from build123d import *

# Parameters (mm, degrees)
BOSS_EXTRUDE1_DEPTH      = 17
SKETCH10_W               = 3
SKETCH10_H               = 4
SKETCH10_H_2             = 2
BOSS_EXTRUDE8_DEPTH      = 0.4
SKETCH11_W               = 2
SKETCH11_H               = 2.1
SKETCH11_W_2             = 4
BOSS_EXTRUDE9_DEPTH      = 0.4
FILLET5_R                = 0.4
SPLIT2_SURFACE_1_BACK    = 26.421
SPLIT2_SURFACE_1_DEPTH   = 52.842
SPLIT2_SURFACE_2_BACK    = 26.421
SPLIT2_SURFACE_2_DEPTH   = 52.842
FILLET6_R                = 1.5
SKETCH13_W               = 5.8
SKETCH13_H               = 8.5
BOSS_EXTRUDE10_DEPTH     = 3
FILLET7_R                = 4
SPLIT3_SURFACE_3_BACK    = 34.598
SPLIT3_SURFACE_3_DEPTH   = 69.196
SPLIT3_SURFACE_4_BACK    = 34.598
SPLIT3_SURFACE_4_DEPTH   = 69.196
CUT_EXTRUDE1_DEPTH       = 1.5
CUT_EXTRUDE2_DEPTH       = 29.664263465
DELETEFACE1_START        = 1.5
DELETEFACE1_DEPTH        = 12
CUT_EXTRUDE3_DEPTH       = 8
MOVE_START               = 1.5
MOVE_FACE1_OUTLINE_W     = 2.5
MOVE_FACE1_OUTLINE_H     = 4
MOVE_FACE1_OUTLINE_H_2   = 2
MOVE_FACE1_DEPTH         = 3
MOVE_FACE1_2_OUTLINE_W   = 0.4
MOVE_FACE1_2_OUTLINE_H   = 2
MOVE_FACE1_2_OUTLINE_H_2 = 4
MOVE_FACE1_2_DEPTH       = 3
MOVE_FACE1_3_OUTLINE_W   = 2.1
MOVE_FACE1_3_OUTLINE_H   = 2
MOVE_FACE1_3_OUTLINE_H_2 = 4
MOVE_FACE1_3_DEPTH       = 0.4
CUT_EXTRUDE4_DEPTH       = 25.456900867
CUT_EXTRUDE4_DEPTH_BACK  = 25.456900867
SPLIT4_SURFACE_5_BACK    = 32.215
SPLIT4_SURFACE_5_DEPTH   = 64.43
SPLIT4_SURFACE_6_BACK    = 32.215
SPLIT4_SURFACE_6_DEPTH   = 64.43
FILLET8_R                = 1
MOVE_START_2             = 1.35
MOVE_FACE2_DEPTH         = 0.15
MOVE_START_3             = 3.2
MOVE_FACE2_2_DEPTH       = 0.15
SPLIT5_START             = -5.8
SPLIT5_OUTLINE_W         = 3
SPLIT5_OUTLINE_H         = 8.5
SPLIT5_DEPTH             = 5.8
SPLIT5_START_2           = 15
SPLIT5_2_OUTLINE_W       = 3
SPLIT5_2_OUTLINE_H       = 8.5
SPLIT5_2_DEPTH           = 5.8
DELETEFACE2_DEPTH        = 1.5
DELETEFACE2_START        = 13.5
DELETEFACE2_2_DEPTH      = 1.5


# Read off the part's stored shape, not the designer's step: DeleteFace1, Move Face1, Move Face2, Split5, DeleteFace2
with BuildPart() as part:
    # Sketch1 → Boss-Extrude1 (new body)
    with BuildSketch(Plane.XY):
        Polygon((0, 0), (1.5, 0), (1.5, 10), (13.5, 10), (13.5, 0), (15, 0), (15, 11.5), (0, 11.5), (0, 10), align=None)
    extrude(amount=BOSS_EXTRUDE1_DEPTH)

    # Sketch10 → Boss-Extrude8 (add)
    with BuildSketch(Plane.XZ.offset(-10)):
        with Locations((12, 14)):
            Rectangle(SKETCH10_W, SKETCH10_H)
        with Locations((12, 10)):
            Rectangle(SKETCH10_W, SKETCH10_H_2)
    boss_extrude8 = extrude(amount=BOSS_EXTRUDE8_DEPTH)

    # Sketch11 → Boss-Extrude9 (add)
    with BuildSketch(Plane.ZY.offset(-13.5)):
        with Locations((10, 8.55)):
            Rectangle(SKETCH11_W, SKETCH11_H)
        with Locations((14, 8.55)):
            Rectangle(SKETCH11_W_2, SKETCH11_H)
    boss_extrude9 = extrude(amount=BOSS_EXTRUDE9_DEPTH)

    # Fillet5
    fillet5_edges = [part.edges().sort_by_distance(p)[0] for p in [
        (13.1, 9.6, 10),
        (13.1, 9.6, 14),
    ]]
    fillet(fillet5_edges, radius=FILLET5_R)


with BuildPart() as body_2:
    # Split2: the piece behind the surface
    add(part.part)
    # Split2 surface: a surface, the sketch's curves swept straight by 52.842 mm
    with BuildLine(Plane.XZ.offset(-SPLIT2_SURFACE_1_BACK), mode=Mode.PRIVATE) as split2_surface_1_path:
        Line((15, 8), (0, 8))
    split2_surface_1 = Shell.extrude(split2_surface_1_path.wire(), (0 * SPLIT2_SURFACE_1_DEPTH, -1 * SPLIT2_SURFACE_1_DEPTH, 0 * SPLIT2_SURFACE_1_DEPTH))
    split(bisect_by=split2_surface_1, keep=Keep.BOTTOM)


with BuildPart() as part_1:
    add(part.part)

    # Split2: split by a surface, the side it looks to stays
    # Split2 surface: a surface, the sketch's curves swept straight by 52.842 mm
    with BuildLine(Plane.XZ.offset(-SPLIT2_SURFACE_2_BACK), mode=Mode.PRIVATE) as split2_surface_2_path:
        Line((15, 8), (0, 8))
    split2_surface_2 = Shell.extrude(split2_surface_2_path.wire(), (0 * SPLIT2_SURFACE_2_DEPTH, -1 * SPLIT2_SURFACE_2_DEPTH, 0 * SPLIT2_SURFACE_2_DEPTH))
    split(bisect_by=split2_surface_2, keep=Keep.TOP)

    # Fillet6
    fillet6_edges = [part_1.edges().sort_by_distance(p)[0] for p in [
        (13.5, 10, 4),
        (1.5, 10, 4),
    ]]
    fillet(fillet6_edges, radius=FILLET6_R)


with BuildPart() as body_2_1:
    add(body_2.part)

    # Combine2: union part
    add(part_1.part)

    # Sketch13 → Boss-Extrude10 (add)
    with BuildSketch(Plane.XZ):
        with Locations((-2.9, 4.25)):
            Rectangle(SKETCH13_W, SKETCH13_H)
        with Locations((17.9, 4.25)):
            Rectangle(SKETCH13_W, SKETCH13_H)
    extrude(amount=-BOSS_EXTRUDE10_DEPTH)

    # Fillet7
    fillet7_edges = [body_2_1.edges().sort_by_distance(p)[0] for p in [
        (20.8, 1.5, 8.5),
        (20.8, 1.5, 0),
        (-5.8, 1.5, 0),
        (-5.8, 1.5, 8.5),
    ]]
    fillet(fillet7_edges, radius=FILLET7_R)


with BuildPart() as body_2_2:
    # Split3: the piece behind the surface
    add(body_2_1.part)
    # Split3 surface: a surface, the sketch's curves swept straight by 69.196 mm
    with BuildLine(Plane.ZY.offset(-SPLIT3_SURFACE_3_BACK), mode=Mode.PRIVATE) as split3_surface_3_path:
        Line((0, 3), (17, 3))
    split3_surface_3 = Shell.extrude(split3_surface_3_path.wire(), (-1 * SPLIT3_SURFACE_3_DEPTH, 0 * SPLIT3_SURFACE_3_DEPTH, 0 * SPLIT3_SURFACE_3_DEPTH))
    split(bisect_by=split3_surface_3, keep=Keep.BOTTOM)

    # Sketch16 → Cut-Extrude1 (cut)
    with BuildSketch(Plane(origin=(0, 3, 0), x_dir=(1, 0, 0), z_dir=(0, 1, 0))):
        Polygon((-1, -7.136751346), (1.5, -5.693375673), (1.5, -2.806624327), (-1, -1.363248654), (-3.5, -2.806624327), (-3.5, -5.693375673), align=None)
        Polygon((16, -1.363248654), (13.5, -2.806624327), (13.5, -5.693375673), (16, -7.136751346), (18.5, -5.693375673), (18.5, -2.806624327), align=None)
    extrude(amount=-CUT_EXTRUDE1_DEPTH, mode=Mode.SUBTRACT)

    # Sketch17 → Cut-Extrude2 (cut, through all)
    with BuildSketch(Plane(origin=(0, 1.5, 0), x_dir=(1, 0, 0), z_dir=(0, 1, 0))):
        with BuildLine():
            Line((16, -5.25), (13.5, -5.25))
            Line((13.5, -5.25), (13.5, -3.25))
            Line((13.5, -3.25), (16, -3.25))
            ThreePointArc((16, -3.25), (17, -4.25), (16, -5.25))
        make_face()
        with BuildLine():
            Line((1.5, -3.25), (1.5, -5.25))
            Line((1.5, -5.25), (-1, -5.25))
            ThreePointArc((-1, -5.25), (-2, -4.25), (-1, -3.25))
            Line((-1, -3.25), (1.5, -3.25))
        make_face()
    extrude(amount=-CUT_EXTRUDE2_DEPTH, mode=Mode.SUBTRACT)


with BuildPart() as body_2_3:
    add(body_2_1.part)

    # Split3: split by a surface, the side it looks to stays
    # Split3 surface: a surface, the sketch's curves swept straight by 69.196 mm
    with BuildLine(Plane.ZY.offset(-SPLIT3_SURFACE_4_BACK), mode=Mode.PRIVATE) as split3_surface_4_path:
        Line((0, 3), (17, 3))
    split3_surface_4 = Shell.extrude(split3_surface_4_path.wire(), (-1 * SPLIT3_SURFACE_4_DEPTH, 0 * SPLIT3_SURFACE_4_DEPTH, 0 * SPLIT3_SURFACE_4_DEPTH))
    split(bisect_by=split3_surface_4, keep=Keep.TOP)

    # Combine3: union body 2 2
    add(body_2_2.part)

    # DeleteFace1 outline → DeleteFace1 (cut)
    with BuildSketch(Plane.YZ.offset(DELETEFACE1_START)):
        Polygon((10, -1), (10, 8), (10, 9), (7, 9), (7, -1), align=None)
    extrude(amount=DELETEFACE1_DEPTH, mode=Mode.SUBTRACT)

    # Mirror1: Boss-Extrude8, Boss-Extrude9 across plane
    add(boss_extrude8.mirror(Plane.ZY.offset(-7.5)))
    add(boss_extrude9.mirror(Plane.ZY.offset(-7.5)))

    # Sketch18 → Cut-Extrude3 (cut)
    with BuildSketch(Plane.XY.offset(16)):
        with BuildLine():
            Line((13.5, 10), (10.5, 10))
            Line((10.5, 10), (10.5, 9.6))
            Line((10.5, 9.6), (12.7, 9.6))
            ThreePointArc((12.7, 9.6), (12.982842712, 9.482842712), (13.1, 9.2))
            Line((13.1, 9.2), (13.1, 7.5))
            Line((13.1, 7.5), (13.5, 7.5))
            Line((13.5, 7.5), (13.5, 10))
        make_face()
    extrude(amount=-CUT_EXTRUDE3_DEPTH, mode=Mode.SUBTRACT)

    # Move Face1 outline → Move Face1 (cut)
    with BuildSketch(Plane.YZ.offset(MOVE_START)):
        with Locations((8.75, 14)):
            Rectangle(MOVE_FACE1_OUTLINE_W, MOVE_FACE1_OUTLINE_H)
        with Locations((8.75, 10)):
            Rectangle(MOVE_FACE1_OUTLINE_W, MOVE_FACE1_OUTLINE_H_2)
    extrude(amount=MOVE_FACE1_DEPTH, mode=Mode.SUBTRACT)

    # Move Face1 2 outline → Move Face1 2 (add)
    with BuildSketch(Plane.YZ.offset(MOVE_START)):
        with Locations((9.8, 2.35)):
            Rectangle(MOVE_FACE1_2_OUTLINE_W, MOVE_FACE1_2_OUTLINE_H)
        with Locations((9.8, 6.35)):
            Rectangle(MOVE_FACE1_2_OUTLINE_W, MOVE_FACE1_2_OUTLINE_H_2)
    extrude(amount=MOVE_FACE1_2_DEPTH)

    # Move Face1 3 outline → Move Face1 3 (add)
    with BuildSketch(Plane.YZ.offset(MOVE_START)):
        with Locations((8.55, 2.35)):
            Rectangle(MOVE_FACE1_3_OUTLINE_W, MOVE_FACE1_3_OUTLINE_H)
        with Locations((8.55, 6.35)):
            Rectangle(MOVE_FACE1_3_OUTLINE_W, MOVE_FACE1_3_OUTLINE_H_2)
    extrude(amount=MOVE_FACE1_3_DEPTH)

    # Sketch19 → Cut-Extrude4 (cut, two sides: drawn at the far end of the back side and taken through both)
    with BuildSketch(Plane.ZY.offset(-7.5).offset(-CUT_EXTRUDE4_DEPTH_BACK)):
        Polygon((11.6, 62.452218571), (11.6, 13.786177198), (11.6, -3.966275857), (11.6, -52.632317231), (108.932082748, -52.632317231), (108.932082748, 62.452218571), align=None)
    extrude(amount=CUT_EXTRUDE4_DEPTH + CUT_EXTRUDE4_DEPTH_BACK, mode=Mode.SUBTRACT)


with BuildPart() as body_2_3_1:
    # Split4: the piece behind the surface
    add(body_2_3.part)
    # Split4 surface: a surface, the sketch's curves swept straight by 64.43 mm
    with BuildLine(Plane.ZY.offset(-7.5).offset(-SPLIT4_SURFACE_5_BACK), mode=Mode.PRIVATE) as split4_surface_5_path:
        Line((9.853674878, 13.930908587), (9.853674878, -3.706091584))
    split4_surface_5 = Shell.extrude(split4_surface_5_path.wire(), (-1 * SPLIT4_SURFACE_5_DEPTH, 0 * SPLIT4_SURFACE_5_DEPTH, 0 * SPLIT4_SURFACE_5_DEPTH))
    split(bisect_by=split4_surface_5, keep=Keep.BOTTOM)


with BuildPart() as body_2_4:
    add(body_2_3.part)

    # Split4: split by a surface, the side it looks to stays
    # Split4 surface: a surface, the sketch's curves swept straight by 64.43 mm
    with BuildLine(Plane.ZY.offset(-7.5).offset(-SPLIT4_SURFACE_6_BACK), mode=Mode.PRIVATE) as split4_surface_6_path:
        Line((9.853674878, 13.930908587), (9.853674878, -3.706091584))
    split4_surface_6 = Shell.extrude(split4_surface_6_path.wire(), (-1 * SPLIT4_SURFACE_6_DEPTH, 0 * SPLIT4_SURFACE_6_DEPTH, 0 * SPLIT4_SURFACE_6_DEPTH))
    split(bisect_by=split4_surface_6, keep=Keep.TOP)

    # Fillet8
    fillet8_edges = [body_2_4.edges().sort_by_distance(p)[0] for p in [
        (1.5, 10, 10.726837439),
        (13.5, 10, 10.726837439),
    ]]
    fillet(fillet8_edges, radius=FILLET8_R)

    # Combine4: union body 2 3
    add(body_2_3_1.part)

    # Move Face2 outline → Move Face2 (cut)
    with BuildSketch(Plane.XY.offset(MOVE_START_2)):
        Polygon((4.5, 10), (1.5, 10), (1.5, 7.5), (1.9, 7.5), (1.9, 9.6), (4.5, 9.6), align=None)
    extrude(amount=MOVE_FACE2_DEPTH, mode=Mode.SUBTRACT)

    # Move Face2 2 outline → Move Face2 2 (cut)
    with BuildSketch(Plane.XY.offset(MOVE_START_3)):
        Polygon((4.5, 10), (1.5, 10), (1.5, 7.5), (1.9, 7.5), (1.9, 9.6), (4.5, 9.6), align=None)
    extrude(amount=MOVE_FACE2_2_DEPTH, mode=Mode.SUBTRACT)

    # Split5 outline → Split5 (cut)
    with BuildSketch(Plane.YZ.offset(SPLIT5_START)):
        with Locations((1.5, 4.25)):
            Rectangle(SPLIT5_OUTLINE_W, SPLIT5_OUTLINE_H)
    extrude(amount=SPLIT5_DEPTH, mode=Mode.SUBTRACT)

    # Split5 2 outline → Split5 2 (cut)
    with BuildSketch(Plane.YZ.offset(SPLIT5_START_2)):
        with Locations((1.5, 4.25)):
            Rectangle(SPLIT5_2_OUTLINE_W, SPLIT5_2_OUTLINE_H)
    extrude(amount=SPLIT5_2_DEPTH, mode=Mode.SUBTRACT)

    # DeleteFace2 outline → DeleteFace2 (add)
    with BuildSketch(Plane.YZ):
        Polygon((0, 3.25), (0, 0), (4, 0), (4, 8), (0, 8), (0, 5.25), align=None)
    extrude(amount=DELETEFACE2_DEPTH)

    # DeleteFace2 2 outline → DeleteFace2 2 (add)
    with BuildSketch(Plane.YZ.offset(DELETEFACE2_START)):
        Polygon((0, 3.25), (0, 0), (4, 0), (4, 8), (0, 8), (0, 5.25), align=None)
    extrude(amount=DELETEFACE2_2_DEPTH)


solid = body_2_4.part
The listing builds one solid part. Answer for the finished solid, in the listing's coordinates (mm). A direction names the side the tool comes from. Give positions to 0.01 mm unless a question says otherwise; leave off trailing zeros. Write each loop counter-clockwise with the first axis right and the second up, starting at its lowest first coordinate (ties: lowest second). Pieces come first, ordered by that corner, then holes. Notation, with made-up numbers: (12.25, 0) -> (48.25, 0) arc R20 cw to (48.25, 28) -> close; hole circle Ø11 at (-31, 15). An arc over 180 degrees is marked (long way). One line per question, with ' | ' between items. Start each with the question number.
1. For faces 1 (the flat face through (2.4, 9.8, 3.2)), 2 (the flat face through (3, 9.6, 2)), 3 (the cylindrical face through (1.785, 9.699, 10.715)), determine the directions among +Z, -Z, +X, -X, +Y, -Y from which every point of the face is accessible in a straight line to the end or side of a thin tool.
2. Section B-B (z = 9.5) is taken. Determine the outline of the cut face in (x, y).
3. For a pull along Z with two mould halves and no side action, classify faces 4 (the cylindrical face through (13.199, 9.715, 10.739)), 5 (the flat face through (2.4, 9.8, 1.5)), 6 (the flat face through (2.3, 9.8, 4.35)) as pulls with the +Z half, pulls with the -Z half, needs draft (parallel to the pull), parting line crosses it, or undercut.
4. Find the intervals of material crossed by probe 1 along X at (y, z) = (1.5, 7.75); probe 2 along Y at (x, z) = (8, 7), in increasing order.
5. Section D-D (z = 1.75) is taken. Determine the outline of the cut face in (x, y).
6. Given pin 1 Ø3 at (x, z) = (3.5, 7) entering from -Y; pin 2 Ø3 at (x, y) = (8, 7.5) entering from -Z, each flat-ended and moving along its own axis, determine where each tip first touches the part or whether it passes through.
7. Section A-A (y = 5.75) is taken. Determine the outline of the cut face in (x, z).
Response values:
1) face 1: -Y | face 2: +Z, -Z, -Y | face 3: +Z, -Y
2) outline: (0, 0) -> (1.5, 0) -> (1.5, 10) -> (13.5, 10) -> (13.5, 0) -> (15, 0) -> (15, 11.5) -> (0, 11.5) -> close
3) face 4: needs draft | face 5: pulls with the -Z half | face 6: undercut
4) probe 1: 0 to 1.5, 13.5 to 15 | probe 2: 10 to 11.5
5) outline: (0, 0) -> (1.5, 0) -> (1.5, 7.5) -> (1.9, 7.5) -> (1.9, 9.6) -> (4.5, 9.6) -> (4.5, 10) -> (13.5, 10) -> (13.5, 0) -> (15, 0) -> (15, 11.5) -> (0, 11.5) -> close
6) pin 1: y = 9.6 | pin 2: through
7) outline: (0, 0) -> (1.5, 0) -> (1.5, 11.6) -> (0, 11.6) -> close; (13.5, 0) -> (15, 0) -> (15, 11.6) -> (13.5, 11.6) -> close
